Part model, mm, in its own coordinate system. Face numbers are marked on the shaded views. A direction names the side the tool comes from. Round coordinates to 2 decimals unless told otherwise and drop trailing zeros. Write each loop counter-clockwise with the first axis right and the second up, starting at its lowest first coordinate (ties: lowest second). Pieces come first, ordered by that corner, then holes. Notation, with made-up numbers: (-18.5, 85.5) -> (14.5, 85.5) arc R25 ccw to (14.5, 112.5) -> close; hole circle Ø2 at (16, 15). An arc over 180 degrees is marked (long way). Use CSV: the item, a comma, the result in double quotes. Start each with the question number.
(1) Saw through at D-D (z = 15.5). Give the cut face in (x, y), plus the area to 3 significant figures.
(2) Two-plate mould, pull along X, no slides. Class the marked faces 6, 7 and 8: released by +X, released by -X, zero draft, split by the parting line, or undercut.
(3) Saw through at C-C (y = 0). Give the cut face in (x, z), plus the area to 3 significant figures.
(4) Which spindle directions (+Z, -Z, +X, -X, +Y, -Y) get a long thin tool onto all of the face, cutting with end or side? Do the marked faces 1, 2, 3, 4 and 5. Say none if no direction does.
(5) Saw through at A-A (z = 1.5). Give the cut face in (x, y), plus the area to 3 significant figures.
(6) Drop flat-ended pins along their axis: pin 1 (3.5 mm diameter, centred on x = 13.5, z = 5.5, fed in from +Y); pin 2 (4 mm diameter, centred on x = 3.5, y = 2.5, fed in from +Z); pin 3 (2.5 mm diameter, centred on y = 1.5, z = 17, fed in from +X). Give the stop position or say it passes through.
(7) Probe line 1 (X direction, y = -11.75, z = 8); line 2 (X direction, y = 8.5, z = 8.25); line 3 (X direction, y = 1.25, z = 11.5). List the from-to ranges inside material, lowest first. Write a range as [from, to].
(8) Saw through at B-B (x = -14). Give the cut face in (y, z), plus the area to 3 significant figures.
Autodesk Inventor part; units mm, degrees
ref_plane "YZ Plane" through (0, 0, 0) normal (1, 0, 0) x (0, 1, 0)
ref_plane "XZ Plane" through (0, 0, 0) normal (0, 1, 0) x (-1, 0, 0)
ref_plane "XY Plane" through (0, 0, 0) normal (0, 0, 1) x (1, 0, 0)
sketch "스케치1" plane through (0, 0, 0) normal (0, 0, 1) x (1, 0, 0)
  line L0 (20.2592, -13.6377) -> (-20.2592, -13.6377)
  line L1 (-20.2592, -13.6377) -> (-20.2592, 13.6377)
  line L2 (-20.2592, 13.6377) -> (20.2592, 13.6377)
  line L3 (20.2592, 13.6377) -> (20.2592, -13.6377)
  line L4 (20.2592, -13.6377) -> (-20.2592, 13.6377) construction
  line L5 (-20.2592, -13.6377) -> (20.2592, 13.6377) construction
  point P0 (0, 0)
extrude "돌출1" add sketch "스케치1" along normal blind 20
sketch "스케치2" plane through (0, 0, 20) normal (0, 0, 1) x (1, 0, 0)
  line L0 (20.2592, 13.6377) -> (-20.2592, 13.6377)
  line L1 (-10.0264, 13.6377) -> (-10.0264, -1.4111)
  line L2 (-20.2592, 13.6377) -> (-20.2592, -13.6377)
  arc A0 (-20.2592, -9.7293) -> (-10.0264, -1.4111) centre (-19.2526, -0.5144) ccw
  line L3 (-10.0264, 13.6377) -> (-20.2592, 13.6377)
  line L4 (-20.2592, -9.7293) -> (-20.2592, 13.6377)
  line L5 (7.8725, 13.6377) -> (20.2592, 13.6377)
  line L6 (20.2592, 13.6377) -> (20.2592, 8.2439)
  line L7 (20.2592, 8.2439) -> (7.8725, 8.2439)
  line L8 (7.8725, 8.2439) -> (7.8725, 13.6377)
  point P0 (0, 0)
extrude "돌출2" cut sketch "스케치2" against normal blind 20
sketch "스케치3" plane through (0, 0, 20) normal (0, 0, 1) x (1, 0, 0)
  line L0 (-10.0264, -1.4111) -> (-10.0264, 13.6377)
  circle A0 centre (-10.0264, 2.161) radius 10.136
  line L1 (20.2592, 8.2439) -> (20.2592, -13.6377)
  line L2 (20.2592, 7.0816) -> (20.2592, -8.6286)
  line L3 (8.5169, 7.0816) -> (8.5169, -0.7735)
  arc A1 (8.5169, -0.7735) -> (20.2592, -8.6286) centre (17.3236, -0.3127) ccw
  line L4 (8.5169, 7.0816) -> (8.5169, 8.2439)
  line L5 (8.5169, 8.2439) -> (20.2592, 8.2439)
  point P0 (0, 0)
extrude "돌출3" cut sketch "스케치3" against normal blind 5 contours A0
extrude "돌출4" cut sketch "스케치3" against normal blind 10 contours L1 A1 L3 L4 L5
sketch "스케치4" plane through (0, 0, 15) normal (0, 0, 1) x (1, 0, 0)
  line L0 (-10.0264, -1.4111) -> (-10.0264, 12.2971)
  circle A0 centre (-10.0264, 2.488) radius 5.4337
  point P0 (0, 0)
extrude "돌출5" add sketch "스케치4" along normal blind 5
sketch "스케치5" plane through (-10.0264, 2.488, 20) normal (0, 0, 1) x (1, 0, 0)
  line L0 (0, -3.8991) -> (0, 5.4337)
  circle A0 centre (0, 0.0967) radius 3.434
  point P0 (10.0264, -2.488)
extrude "돌출6" add sketch "스케치5" along normal blind 2
sketch "스케치6" plane through (0, 0, 10) normal (0, 0, 1) x (1, 0, 0)
  line L0 (20.2592, 8.2439) -> (20.2592, -13.6377)
  circle A0 centre (20.2592, 0) radius 5.9354
  point P0 (0, 0)
extrude "돌출7" cut sketch "스케치6" against normal blind 20
sketch "스케치7" plane through (0, 0, 20) normal (0, 0, 1) x (1, 0, 0)
  line L0 (20.2592, -13.6377) -> (-20.2592, -13.6377)
  line L1 (-1.3274, -10.3147) -> (6.1983, -10.3147)
  line L2 (6.1983, -10.3147) -> (6.1983, -13.6377)
  line L3 (6.1983, -13.6377) -> (-1.3274, -13.6377)
  line L4 (-1.3274, -13.6377) -> (-1.3274, -10.3147)
  point P0 (0, 0)
extrude "돌출8" cut sketch "스케치7" against normal blind 20
properties part number "240626_part1"
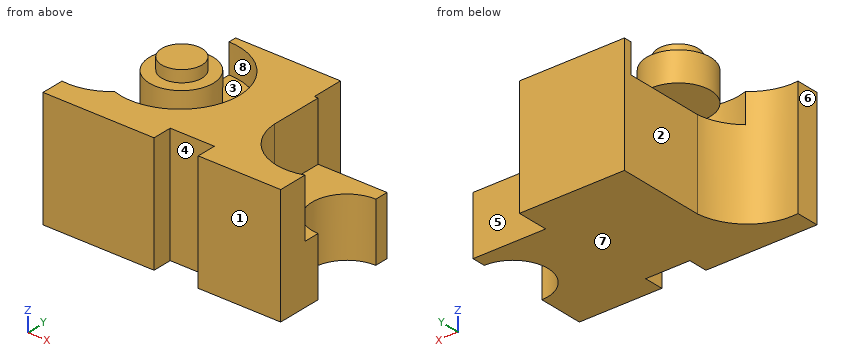
Answers:
1,outline,"(-20.26, -13.64) -> (-1.33, -13.64) -> (-1.33, -10.31) -> (6.2, -10.31) -> (6.2, -13.64) -> (20.26, -13.64) -> (20.26, -8.63) arc R8.82 cw to (8.52, -0.77) -> (8.52, 8.24) -> (7.87, 8.24) -> (7.87, 13.64) -> (-10.03, 13.64) -> (-10.03, 12.3) arc R10.14 cw (long way) to (-13.14, -7.48) arc R9.27 cw to (-20.26, -9.73) -> close; circle Ø10.87 at (-10.03, 2.49)"
1,area,"529 mm²"
2,face 6,"released by -X"
2,face 7,"zero draft"
2,face 8,"undercut"
3,outline,"(-14.86, 15) -> (-10.03, 15) -> (-10.03, 0) -> (14.32, 0) -> (14.32, 10) -> (8.52, 10) -> (8.52, 20) -> (-0.12, 20) -> (-0.12, 15) -> (-5.2, 15) -> (-5.2, 20) -> (-7.77, 20) -> (-7.77, 22) -> (-12.29, 22) -> (-12.29, 20) -> (-14.86, 20) -> close"
3,area,"437 mm²"
4,face 1,"+Z, -Z, +X, -X, -Y"
4,face 2,"-Z, -X, +Y"
4,face 3,"+Z"
4,face 4,"+Z, -Z, -Y"
4,face 5,"+Z, -Z, +X, +Y"
5,outline,"(-20.26, -13.64) -> (-1.33, -13.64) -> (-1.33, -10.31) -> (6.2, -10.31) -> (6.2, -13.64) -> (20.26, -13.64) -> (20.26, -5.94) arc R5.94 cw to (20.26, 5.94) -> (20.26, 8.24) -> (7.87, 8.24) -> (7.87, 13.64) -> (-10.03, 13.64) -> (-10.03, -1.41) arc R9.27 cw to (-20.26, -9.73) -> close"
5,area,"736 mm²"
6,pin 1,"stops at y = 8.24"
6,pin 2,"stops at z = 20"
6,pin 3,"stops at x = 8.52"
7,line 1,"x = [-20.26, -1.33], [6.2, 20.26]"
7,line 2,"x = [-10.03, 7.87]"
7,line 3,"x = [-10.03, 8.52]"
8,outline,"(-13.64, 0) -> (-8.15, 0) -> (-8.15, 20) -> (-13.64, 20) -> close; (-1.22, 15) -> (6.19, 15) -> (6.19, 20) -> (-1.22, 20) -> close"
8,area,"147 mm²"
